Autodesk Inventor part; units mm, degrees
ref_plane "YZ Plane" through (0, 0, 0) normal (1, 0, 0) x (0, 1, 0)
ref_plane "XZ Plane" through (0, 0, 0) normal (0, 1, 0) x (-1, 0, 0)
ref_plane "XY Plane" through (0, 0, 0) normal (0, 0, 1) x (1, 0, 0)
sketch "Sketch1" plane through (0, 0, 0) normal (0, 0, 1) x (1, 0, 0)
  line L0 (0, 0) -> (28, 0)
  line L1 (28, 0) -> (28, 28)
  line L2 (28, 28) -> (0, 28)
  line L3 (0, 28) -> (0, 0)
  dimension "d0" = 28
  dimension "d1" = 28
extrude "Extrusion1" add sketch "Sketch1" along normal blind 8
fillet "Fillet1" radius 1.5 4 edges at (0, 0, 4) (28, 0, 4) (0, 28, 4) (28, 28, 4)
sketch "Sketch3" plane through (0, 0, 8) normal (0, 0, 1) x (1, 0, 0)
  line L0 (1.5, 28) -> (26.5, 28)
  line L1 (0, 1.5) -> (0, 26.5)
  line L2 (26.5, 0) -> (1.5, 0)
  line L3 (28, 26.5) -> (28, 1.5)
  point P0 (2.5, 2.5)
  point P1 (25.5, 2.5)
  point P2 (2.5, 25.5)
  point P3 (25.5, 25.5)
  dimension "d10" = 2.5
  dimension "d11" = 2.5
  dimension "d12" = 2.5
  dimension "d13" = 2.5
  dimension "d14" = 2.5
  dimension "d15" = 2.5
  dimension "d16" = 2.5
  dimension "d17" = 2.5
hole "Hole1" at (2.5, 2.5, 8) at (25.5, 2.5, 8) at (2.5, 25.5, 8) at (25.5, 25.5, 8) direction (0, 0, -1) diameter 2.5 end through all
properties part number "stepper_middle_28"
Read the model definition and answer for the solid it produces. Units are mm, in the model's axes. Coordinates: 2 decimals unless noted, no trailing zeros. Write each loop counter-clockwise with the first axis right and the second up, starting at its lowest first coordinate (ties: lowest second). Pieces come first, ordered by that corner, then holes. Notation, with made-up numbers: (66.5, 51) - (106.5, 51) arc R27 cw to (106.5, 86) - close; hole circle Ø7 at (25.5, 30). An arc over 180 degrees is marked (long way). Answer as a JSON object with one key per item and string values. Group by question number.
1. The mould has two halves that part along X. Classify faces 1 (the flat face through (14, 0, 4)), 2 (the cylindrical face through (26.72, 2.77, 3.94)), 3 (the cylindrical face through (27.57, 27.55, 4.06)), 4 (the flat face through (0, 14, 4)): +X half, -X half, draft (parallel to the pull), parting line (faces both ways), or undercut.
2. A cutting plane is placed at A-A (x = 25.5). Determine the outline of the cut face in (y, z), plus the area to 3 significant figures.
3. A cutting plane is placed at C-C (z = 3.75). Determine the outline of the cut face in (x, y).
4. Consider L1, parallel to X at y = 2.5, z = 4.5; L2, parallel to Y at x = 3, z = 4. Determine where each line is inside the solid, lowest interval first. Write a range as [from, to].
Worked out:
{
 "1": {"face 1": "draft", "face 2": "undercut", "face 3": "+X half", "face 4": "-X half"},
 "2": {"outline": "(0, 0) - (1.25, 0) - (1.25, 8) - (0, 8) - close; (3.75, 0) - (24.25, 0) - (24.25, 8) - (3.75, 8) - close; (26.75, 0) - (28, 0) - (28, 8) - (26.75, 8) - close", "area": "184 mm²"},
 "3": {"outline": "(0, 1.5) arc R1.5 ccw to (1.5, 0) - (26.5, 0) arc R1.5 ccw to (28, 1.5) - (28, 26.5) arc R1.5 ccw to (26.5, 28) - (1.5, 28) arc R1.5 ccw to (0, 26.5) - close; hole circle Ø2.5 at (2.5, 2.5); hole circle Ø2.5 at (2.5, 25.5); hole circle Ø2.5 at (25.5, 2.5); hole circle Ø2.5 at (25.5, 25.5)"},
 "4": {"L1": "x = [0, 1.25], [3.75, 24.25], [26.75, 28]", "L2": "y = [0, 1.35], [3.65, 24.35], [26.65, 28]"}
}
